Source: CAD feature listing. Evaluate the final solid. Frame: model axes, mm. A direction names the side the tool comes from. Give positions to 0.01 mm unless a question says otherwise; leave off trailing zeros. Write each loop counter-clockwise with the first axis right and the second up, starting at its lowest first coordinate (ties: lowest second). Pieces come first, ordered by that corner, then holes. Notation, with made-up numbers: M 0,65.25 L 51,65.25 A20 ccw 51,70.25 Z; hole C 52,86.5 d7. An arc over 180 degrees is marked long. Return JSON: item names as keys, results as strings.
```python
from build123d import *

# Parameters (mm, degrees)
F1_DEPTH  = 15
F2_T      = -2
F3_R      = 1.5
F4_DEPTH  = 2
F5_R      = 1.5
F6_DEPTH  = 13
F7_W      = 5
F7_H      = 2
F8_DEPTH  = 2
F9_R      = 1.5
F10_DEPTH = 2
F11_R     = 1
F12_DEPTH = 7


with BuildPart() as f1:
    # F0 (on Top) → F1 (new body)
    with BuildSketch(Plane.XY):
        with BuildLine():
            Line((-40.5, 35.5), (-40.5, 14.5))
            Line((-40.5, 14.5), (-40.5, -14.5))
            ThreePointArc((-40.5, -14.5), (-39.6213203436, -16.6213203436), (-37.5, -17.5))
            Line((-37.5, -17.5), (-12.5, -17.5))
            ThreePointArc((-12.5, -17.5), (-10.3786796564, -18.3786796564), (-9.5, -20.5))
            Line((-9.5, -20.5), (-9.5, -42.5))
            ThreePointArc((-9.5, -42.5), (-8.6213203436, -44.6213203436), (-6.5, -45.5))
            Line((-6.5, -45.5), (55.5, -45.5))
            ThreePointArc((55.5, -45.5), (57.6213203436, -44.6213203436), (58.5, -42.5))
            Line((58.5, -42.5), (58.5, 35.5))
            ThreePointArc((58.5, 35.5), (57.6213203436, 37.6213203436), (55.5, 38.5))
            Line((55.5, 38.5), (-37.5, 38.5))
            ThreePointArc((-37.5, 38.5), (-39.6213203436, 37.6213203436), (-40.5, 35.5))
        make_face()
    extrude(amount=F1_DEPTH)

    # F2
    f2_openings = [f1.faces().sort_by_distance(p)[0] for p in [
        (12.966173, -0.233802, 15),
    ]]
    offset(amount=F2_T, openings=f2_openings)

    # F3 (on face) → F4 (cut, through all)
    with BuildSketch(Plane.XY.offset(2)):
        with Locations((-29, 11.5)):
            Circle(F3_R)
        with Locations((29, 11.5)):
            Circle(F3_R)
        with Locations((-29, -11.5)):
            Circle(F3_R)
        with Locations((29, -11.5)):
            Circle(F3_R)
    extrude(amount=-F4_DEPTH, mode=Mode.SUBTRACT)

    # F5 (on face) → F6 (join, through all)
    with BuildSketch(Plane.XY.offset(2)):
        with BuildLine():
            Line((-2.5, -43.5), (-2.5, -41))
            Line((-2.5, -41), (-2.5, -20.5))
            ThreePointArc((-2.5, -20.5), (-3.9644660941, -16.9644660941), (-7.5, -15.5))
            Line((-7.5, -15.5), (-12.5, -15.5))
            Line((-12.5, -15.5), (-7.5, -20.5))
            Line((-7.5, -20.5), (-7.5, -38.5))
            Line((-7.5, -38.5), (-7.5, -43.5))
            Line((-7.5, -43.5), (-2.5, -43.5))
        make_face()
        with Locations((-5, -41)):
            Circle(F5_R, mode=Mode.SUBTRACT)
        with BuildLine():
            ThreePointArc((54, -38.5), (52.232233047, -39.232233047), (51.5, -41))
            Line((51.5, -41), (51.5, -43.5))
            Line((51.5, -43.5), (56.5, -43.5))
            Line((56.5, -43.5), (56.5, -38.5))
            Line((56.5, -38.5), (54, -38.5))
        make_face()
        with Locations((54, -41)):
            Circle(F5_R, mode=Mode.SUBTRACT)
        with BuildLine():
            ThreePointArc((51.5, 34), (52.232233047, 32.232233047), (54, 31.5))
            Line((54, 31.5), (56.5, 31.5))
            Line((56.5, 31.5), (56.5, 36.5))
            Line((56.5, 36.5), (51.5, 36.5))
            Line((51.5, 36.5), (51.5, 34))
        make_face()
        with Locations((54, 34)):
            Circle(F5_R, mode=Mode.SUBTRACT)
        with BuildLine():
            Line((-38.5, 31.5), (-36, 31.5))
            ThreePointArc((-36, 31.5), (-34.232233047, 32.232233047), (-33.5, 34))
            Line((-33.5, 34), (-33.5, 36.5))
            Line((-33.5, 36.5), (-38.5, 36.5))
            Line((-38.5, 36.5), (-38.5, 31.5))
        make_face()
        with Locations((-36, 34)):
            Circle(F5_R, mode=Mode.SUBTRACT)
    extrude(amount=F6_DEPTH)

    # F7 (on Top) → F8 (cut, through all)
    with BuildSketch(Plane.XY):
        with Locations((-14, 33)):
            Rectangle(F7_W, F7_H)
        with Locations((41, 33)):
            Rectangle(F7_W, F7_H)
        with Locations((41, 15)):
            Rectangle(F7_W, F7_H)
        with Locations((-14, 15)):
            Rectangle(F7_W, F7_H)
        with Locations((25, -27.5)):
            Rectangle(F7_W, F7_H)
        with Locations((25, -33.5)):
            Rectangle(F7_W, F7_H)
        with Locations((35, -27.5)):
            Rectangle(F7_W, F7_H)
        with Locations((35, -33.5)):
            Rectangle(F7_W, F7_H)
        with Locations((45, -27.5)):
            Rectangle(F7_W, F7_H)
        with Locations((45, -33.5)):
            Rectangle(F7_W, F7_H)
    extrude(amount=F8_DEPTH, mode=Mode.SUBTRACT)

    # F9 (on face) → F10 (cut, through all)
    with BuildSketch(Plane.XY.offset(2)):
        with Locations((54, 34)):
            Circle(F9_R)
        with Locations((-36, 34)):
            Circle(F9_R)
        with Locations((-5, -41)):
            Circle(F9_R)
        with Locations((54, -41)):
            Circle(F9_R)
    extrude(amount=-F10_DEPTH, mode=Mode.SUBTRACT)

    # F11 (on face) → F12 (cut, through all)
    with BuildSketch(Plane(origin=(-9.5, 0, 0), x_dir=(0, -1, 0), z_dir=(-1, 0, 0))):
        with Locations((26.5, 15)):
            Circle(F11_R)
        with Locations((36.5, 15)):
            Circle(F11_R)
    extrude(amount=-F12_DEPTH, mode=Mode.SUBTRACT)


solid = f1.part
```
1) Cut plane D-D, the plane x = -5. Return the cut outline in (y, z), then the cut area to 3 significant figures.
Numbers:
{"outline": "M -45.5,0 L -42.5,0 L -42.5,15 L -45.5,15 Z; M -39.5,0 L 38.5,0 L 38.5,15 L 36.5,15 L 36.5,2 L -16.17,2 L -16.17,15 L -25.5,15 A1 cw -27.5,15 L -35.5,15 A1 cw -37.5,15 L -39.5,15 Z", "area": "527 mm²"}
2) Draft query along X for faces 1 (the face through (27.5, -28, 1)), 2 (the face through (45, -26.5, 1)), 3 (the face through (-6, -36.5, 14)), 4 (the face through (-39.64, -16.6, 7.4)). Return one class per face: released by +X, released by -X, zero draft, split by the parting line, or undercut.
Numbers:
{"face 1": "undercut", "face 2": "undercut", "face 3": "zero draft", "face 4": "released by -X"}
3) Line query: line 1 (Y direction, x = 54, z = 5.25); line 2 (Y direction, x = -20, z = 11); line 3 (Y direction, x = -36, z = 7). Output: solid intervals per line, ascending. Write a range as [from, to].
Numbers:
{"line 1": "y = [-45.5, -42.5], [-39.5, -38.5], [31.5, 32.5], [35.5, 38.5]", "line 2": "y = [-17.5, -15.5], [36.5, 38.5]", "line 3": "y = [-17.5, -15.5], [31.5, 32.5], [35.5, 38.5]"}
4) Cut plane A-A, the plane y = -11.5. Return the cut outline in (x, z).
Numbers:
{"outline": "M -40.5,0 L -30.5,0 L -30.5,2 L -38.5,2 L -38.5,15 L -40.5,15 Z; M -27.5,0 L 27.5,0 L 27.5,2 L -27.5,2 Z; M 30.5,0 L 58.5,0 L 58.5,15 L 56.5,15 L 56.5,2 L 30.5,2 Z"}
5) Cut plane B-B, the plane z = 4. Give the number of separate pieces and of enclosed holes in the cut face, then the cut area to 3 significant figures.
Numbers:
{"separate pieces": "1", "enclosed holes": "5", "area": "886 mm²"}
6) Set-up query: faces 5 (the face through (-11.5, 33, 1)), 6 (the face through (-3.93, -17, 8.41)), 7 (the face through (8, -3, 0)). Return all of +Z, -Z, +X, -X, +Y, -Y with unobstructed straight access to the full face (end or side cutting, diameter ignored); none if empty.
Numbers:
{"face 5": "+Z, -Z", "face 6": "+Z", "face 7": "-Z, +X, -X, +Y, -Y"}
7) Contact query for flat-ended pins moving along their axis: pin 1 Ø6 at (y, z) = (-21.5, 13.5) entering from -X; pin 2 Ø1.2 at (y, z) = (-42, 7) entering from -X. Output: stop coordinate, or through.
Numbers:
{"pin 1": "stops at x = -10.26", "pin 2": "stops at x = -9.5"}
8) Cut plane C-C, the plane x = 20. Return the cut outline in (y, z).
Numbers:
{"outline": "M -45.5,0 L 38.5,0 L 38.5,15 L 36.5,15 L 36.5,2 L -43.5,2 L -43.5,15 L -45.5,15 Z"}
